Design review of the part built by this model. Coordinates are the model's own, in mm. Face numbers are marked on the shaded views. A direction names the side the tool comes from. Coordinates: 2 decimals unless noted, no trailing zeros. Loops run counter-clockwise (first coordinate to the right, second up) from the corner with the lowest first, then second, coordinate; pieces in that order, holes last. Notation, with made-up numbers: (-16.75, 73.5) - (42.25, 73.5) arc R21 ccw to (42.25, 98.5) - close; hole circle Ø3 at (46.25, 7). An arc over 180 degrees is marked (long way). One line per question, with ' | ' between items.
from build123d import *

# Parameters (mm, degrees)
F0_W     = 220
F0_H     = 200
F1_DEPTH = 305
F2_T     = -4
F3_W     = 100
F3_H     = 30
F4_DEPTH = 305.001


with BuildPart() as f1:
    # F0 (on Front) → F1 (new body)
    with BuildSketch(Plane.XZ):
        with Locations((110, 100)):
            Rectangle(F0_W, F0_H)
    extrude(amount=F1_DEPTH)

    # F2
    f2_openings = [f1.faces().sort_by_distance(p)[0] for p in [
        (110, -152.5, 200),
    ]]
    offset(amount=F2_T, openings=f2_openings)

    # F3 (on face) → F4 (cut, through all)
    with BuildSketch(Plane.XZ.offset(305)):
        with Locations((110, 160)):
            Rectangle(F3_W, F3_H)
    extrude(amount=-F4_DEPTH, mode=Mode.SUBTRACT)


solid = f1.part
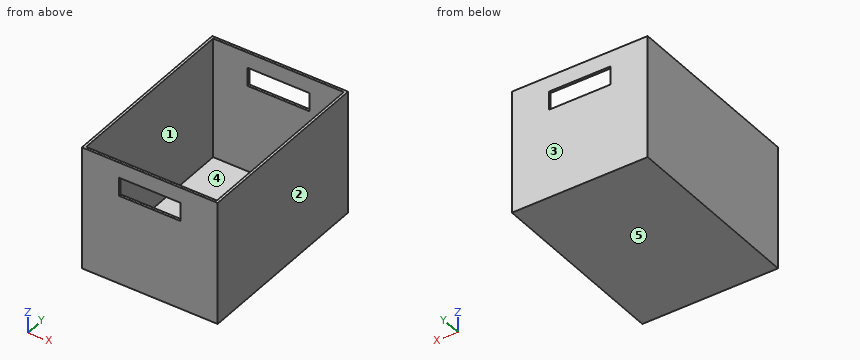
Q1. To check wall thickness, follow line 1 along Y through (x, z) = (159, 88); line 2 along X through (y, z) = (-176, 79); line 3 along Z through (x, y) = (208, -137.5). State the ranges of each line that lie inside material, in increasing order.
Returned:
line 1: y = -305 to -301, -4 to 0 | line 2: x = 0 to 4, 216 to 220 | line 3: z = 0 to 4
Q2. Draft analysis for pull direction X (two halves, no side actions). For the marked faces 1, 2 and 3, state which applies: +X half, -X half, draft (parallel to the pull), parting line (faces both ways), or undercut.
Returned:
face 1: undercut | face 2: +X half | face 3: draft
Q3. Take a section at A-A (z = 158.5). Give the boundary of the cut face in (x, y), plus the area to 3 significant figures.
Returned:
outline: (0, -305) - (60, -305) - (60, -301) - (4, -301) - (4, -4) - (60, -4) - (60, 0) - (0, 0) - close; (160, -305) - (220, -305) - (220, 0) - (160, 0) - (160, -4) - (216, -4) - (216, -301) - (160, -301) - close | area: 3,340 mm²
Q4. Take a section at C-C (z = 99). Give the boundary of the cut face in (x, y).
Returned:
outline: (0, -305) - (220, -305) - (220, 0) - (0, 0) - close; hole (4, -301) - (216, -301) - (216, -4) - (4, -4) - close
Q5. Tool access review of the marked faces 4 and 5: name each direction out of +Z, -Z, +X, -X, +Y, -Y from which nothing blocks a thin tool from reaching the whole face with its end or side.
Returned:
face 4: +Z | face 5: -Z, +X, -X, +Y, -Y
Q6. Take a section at B-B (x = 128). Give the boundary of the cut face in (y, z).
Returned:
outline: (-305, 0) - (0, 0) - (0, 145) - (-4, 145) - (-4, 4) - (-301, 4) - (-301, 145) - (-305, 145) - close; (-305, 175) - (-301, 175) - (-301, 200) - (-305, 200) - close; (-4, 175) - (0, 175) - (0, 200) - (-4, 200) - close
Q7. Take a section at D-D (y = -279). Give the boundary of the cut face in (x, z), plus the area to 3 significant figures.
Returned:
outline: (0, 0) - (220, 0) - (220, 200) - (216, 200) - (216, 4) - (4, 4) - (4, 200) - (0, 200) - close | area: 2,450 mm²
